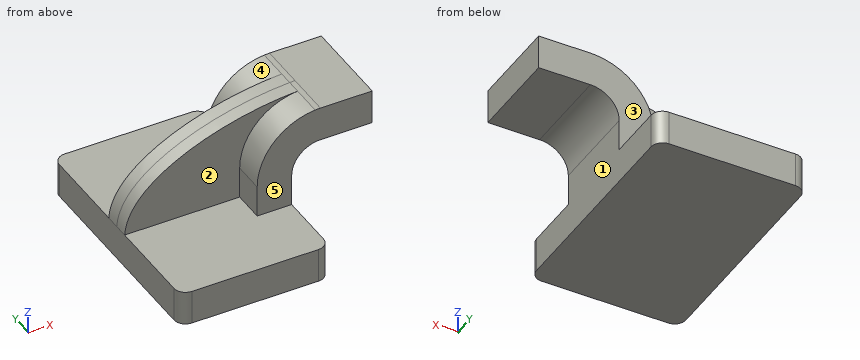
from build123d import *

# Parameters (mm, degrees)
F1_DEPTH = 63.5
F0_W     = 25.4
F0_H     = 19.05
F2_DEPTH = 25.4
F3_DEPTH = 7.9375
F4_R     = 6.35


with BuildPart() as f1:
    # F0 (on Front) → F1 (new body, symmetric)
    with BuildSketch(Plane.XZ):
        Polygon((-41.275, -9.525), (41.275, -9.525), (41.275, 9.525), (22.225, 9.525), (-41.275, 9.525), align=None)
    extrude(amount=F1_DEPTH, both=True)

    # F0 (on Front) → F2 (join, symmetric)
    with BuildSketch(Plane.XZ):
        with BuildLine():
            Line((22.225, 9.525), (41.275, 9.525))
            Line((41.275, 9.525), (41.275, 27.0002))
            ThreePointArc((41.275, 27.0002), (45.9246798487, 38.2255201513), (57.15, 42.8752))
            Line((57.15, 42.8752), (60.325, 42.8752))
            Line((60.325, 42.8752), (60.325, 61.9252))
            Line((60.325, 61.9252), (57.15, 61.9252))
            add(Edge.make_bspline(
                [(54.2163315583, 61.8017691381), (55.1991693528, 61.8523831692), (56.1772996051, 61.8935558804), (57.15, 61.9252)],
                knots=[108.9789344494, 108.9789344494, 108.9789344494, 108.9789344494, 111.5045361635, 111.5045361635, 111.5045361635, 111.5045361635], degree=3))
            ThreePointArc((54.2163315583, 61.8017691381), (31.4379989564, 50.6359489269), (22.225, 27.0002))
            Line((22.225, 27.0002), (22.225, 9.525))
        make_face()
        with Locations((73.025, 52.4002)):
            Rectangle(F0_W, F0_H)
    extrude(amount=F2_DEPTH, both=True)

    # F0 (on Front) → F3 (join, symmetric)
    with BuildSketch(Plane.XZ):
        with BuildLine():
            add(Edge.make_bspline(
                [(-41.275, 9.525), (-39.3669167173, 39.8550550116), (11.8071840745, 59.6177893167), (54.2163315583, 61.8017691381)],
                knots=[0, 0, 0, 0, 108.9789344494, 108.9789344494, 108.9789344494, 108.9789344494], degree=3))
            Line((-41.275, 9.525), (22.225, 9.525))
            Line((22.225, 9.525), (22.225, 27.0002))
            ThreePointArc((22.225, 27.0002), (31.4379989564, 50.6359489269), (54.2163315583, 61.8017691381))
        make_face()
    extrude(amount=F3_DEPTH, both=True)

    # F4
    f4_edges = [f1.edges().sort_by_distance(p)[0] for p in [
        (41.275, -63.5, 0),
        (-41.275, -63.5, 0),
        (41.275, 63.5, 0),
        (-41.275, 63.5, 0),
    ]]
    fillet(f4_edges, radius=F4_R)


solid = f1.part
The listing builds one solid part. Answer for the finished solid, in the listing's coordinates (mm). Face numbers are marked on the shaded views. A direction names the side the tool comes from. Coordinates: 2 decimals unless noted, no trailing zeros. Write each loop counter-clockwise with the first axis right and the second up, starting at its lowest first coordinate (ties: lowest second). Pieces come first, ordered by that corner, then holes. Notation, with made-up numbers: M -24,0 L 4,0 A21 cw 4,18 Z; hole C 37.5,80 d7. An arc over 180 degrees is marked long. Write each question's results on one line, items separated by ' | '.
Item 1: Consider probe 1 along Y at (x, z) = (68, 45.5); probe 2 along Y at (x, z) = (-16, 10); probe 3 along X at (y, z) = (-51.5, -3) (3 decimals). Determine where each line is inside the solid, lowest interval first. Write a range as [from, to].
Answer below:
probe 1: [-25.4, 25.4] | probe 2: [-7.94, 7.94] | probe 3: [-41.275, 41.275]
Item 2: The part is cut by section C-C on y = -45. Determine the outline of the cut face in (x, z) (3 decimals), and give its area (3 significant figures).
Answer below:
outline: M -41.275,-9.525 L 41.275,-9.525 L 41.275,9.525 L -41.275,9.525 Z | area: 1,570 mm2
Item 3: Which of the six approach directions +Z, -Z, +X, -X, +Y, -Y give full straight-line access (tool end or side, diameter ignored) to the marked faces 1, 2, 3, 4 and 5?
Answer below:
face 1: -Z, +X, +Y, -Y | face 2: +Z, -X, -Y | face 3: +Z, +X, -X, +Y | face 4: +Z, -X, +Y | face 5: +Z, +X, -X, -Y
Item 4: The part is cut by section A-A on z = 1.5. Determine the outline of the cut face in (x, y) (3 decimals), and give its area (3 significant figures).
Answer below:
outline: M -41.275,-57.15 A6.35 ccw -34.925,-63.5 L 34.925,-63.5 A6.35 ccw 41.275,-57.15 L 41.275,57.15 A6.35 ccw 34.925,63.5 L -34.925,63.5 A6.35 ccw -41.275,57.15 Z | area: 10,400 mm2
Item 5: Given P1, Ø8.5, axis at x = 66.5, y = -11.5, coming from the -Z side; P2, Ø5, axis at y = 13, z = 22, coming from the -X side (3 decimals); P3, Ø15.5, axis at x = 23, z = 27, coming from the +Y side, each flat-ended and moving along its own axis, determine where each tip first touches the part or whether it passes through.
Answer below:
P1: z = 42.88 | P2: x = 22.225 | P3: y = 25.4
Item 6: The part is cut by section B-B on x = 64. Determine the outline of the cut face in (y, z), and give its area (3 significant figures).
Answer below:
outline: M -25.4,42.88 L 25.4,42.88 L 25.4,61.93 L -25.4,61.93 Z | area: 968 mm2
